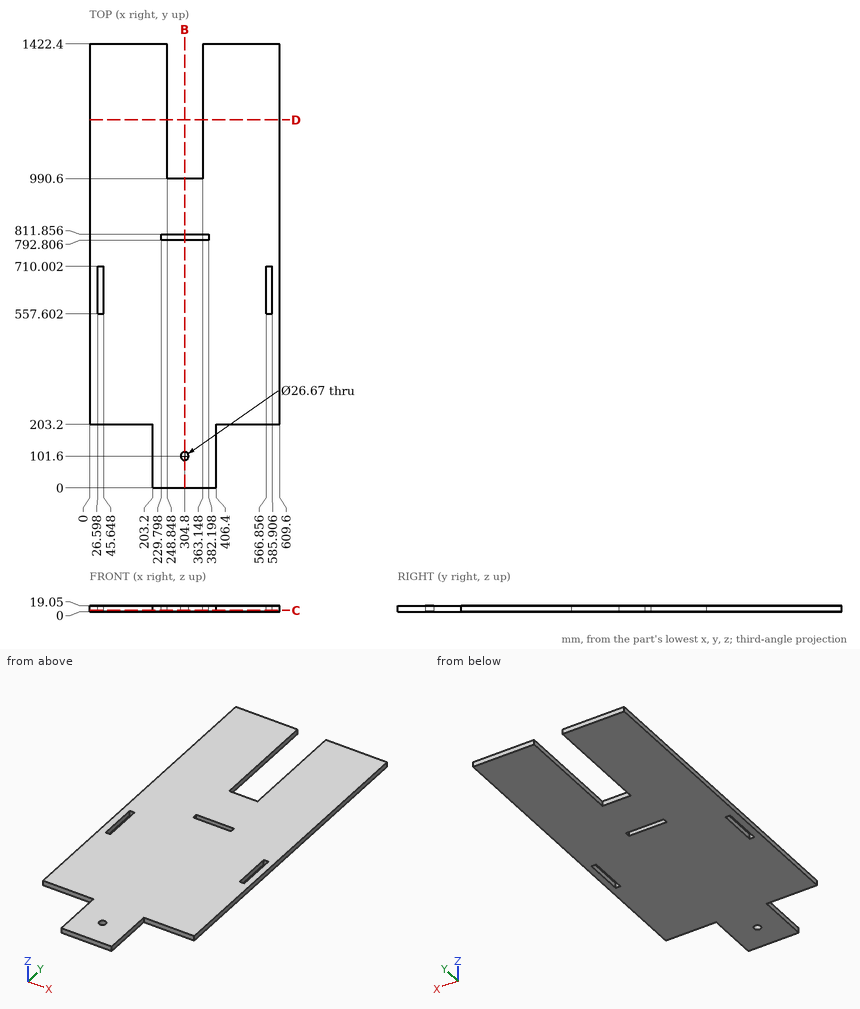
The drawing under review shows one solid part. Ordinate dimensions are in mm from its lowest x, y, z. Give positions to 0.01 mm unless a question says otherwise; leave off trailing zeros. Write each loop counter-clockwise with the first axis right and the second up, starting at its lowest first coordinate (ties: lowest second). Pieces come first, ordered by that corner, then holes. Notation, with made-up numbers: (76, -2.5) -> (121, -2.5) arc R24 ccw to (121, 24.5) -> close; hole circle Ø5 at (81, -14.75). An arc over 180 degrees is marked (long way). Put each result on its own line as item: value.
(1) We need section D-D, the plane y = 1179.5. Give the boundary of the cut face in (x, z).
Results are:
outline: (0, 0) -> (248.85, 0) -> (248.85, 19.05) -> (0, 19.05) -> close; (363.15, 0) -> (609.6, 0) -> (609.6, 19.05) -> (363.15, 19.05) -> close
(2) We need section C-C, the plane z = 4. Give the boundary of the cut face in (x, y) (1 decimal).
Results are:
outline: (0, 203.2) -> (203.2, 203.2) -> (203.2, 0) -> (406.4, 0) -> (406.4, 203.2) -> (609.6, 203.2) -> (609.6, 1422.4) -> (363.1, 1422.4) -> (363.1, 990.6) -> (248.8, 990.6) -> (248.8, 1422.4) -> (0, 1422.4) -> close; hole (26.6, 557.6) -> (45.6, 557.6) -> (45.6, 710) -> (26.6, 710) -> close; hole (229.8, 792.8) -> (382.2, 792.8) -> (382.2, 811.9) -> (229.8, 811.9) -> close; hole circle Ø26.7 at (304.8, 101.6); hole (566.9, 557.6) -> (585.9, 557.6) -> (585.9, 710) -> (566.9, 710) -> close
(3) To check wall thickness, follow probe 1 along Y at (x, z) = (304.8, 4.5) (1 decimal); probe 2 along X at (y, z) = (567.5, 10) (1 decimal); probe 3 along X at (y, z) = (101.6, 9.75) (1 decimal). State the ranges of each line that lie inside material, in increasing order. Write a range as from..to.
Results are:
probe 1: 0..88.3, 114.9..792.8, 811.9..990.6
probe 2: 0..26.6, 45.6..566.9, 585.9..609.6
probe 3: 203.2..291.5, 318.1..406.4
(4) We need section B-B, the plane x = 304.8. State how many separate pieces and enclosed holes the cut face has, and give its area (3 significant figures).
Results are:
separate pieces: 3
enclosed holes: 0
area: 18,000 mm²
(5) For pin 1 Ø8 at (x, z) = (79.5, 13) entering from -Y; pin 2 Ø9.5 at (y, z) = (110.5, 10.5) entering from +X, all flat-tipped, find the tip position at first contact; note any pin that passes through.
Results are:
pin 1: y = 203.2
pin 2: x = 406.4
